Build history of the part. All positions in model axes, mm. Give positions to 0.01 mm unless a question says otherwise; leave off trailing zeros. Loops run counter-clockwise (first coordinate to the right, second up) from the corner with the lowest first, then second, coordinate; pieces in that order, holes last. Notation, with made-up numbers: (2.5, -16.5) -> (46.5, -16.5) arc R26 ccw to (46.5, 7.5) -> close; hole circle Ø5 at (85.25, -13). An arc over 180 degrees is marked (long way). Answer in a Markdown table with one row per item. Add a question column.
from build123d import *

# Parameters (mm, degrees)
F0_R     = 67
F0_R_2   = 8
F0_R_3   = 29.5
F1_DEPTH = 5


with BuildPart() as f1:
    # F0 (on Top) → F1 (new body)
    with BuildSketch(Plane.XY):
        Circle(F0_R)
        with Locations((-15.796341, -47.077298)):
            Circle(F0_R_2, mode=Mode.SUBTRACT)
        with Locations((39.546341, -29.09537)):
            Circle(F0_R_2, mode=Mode.SUBTRACT)
        with Locations((-50, 0)):
            Circle(F0_R_2, mode=Mode.SUBTRACT)
        with Locations((-15.796341, 47.077298)):
            Circle(F0_R_2, mode=Mode.SUBTRACT)
        Circle(F0_R_3, mode=Mode.SUBTRACT)
        with Locations((39.546341, 29.09537)):
            Circle(F0_R_2, mode=Mode.SUBTRACT)
    extrude(amount=F1_DEPTH)


solid = f1.part
(1) Saw through at D-D, the plane y = 33. List the corners of the cut face in (x, z).
(2) Wall check: line 1 along Y through (x, z) = (0, 1.3); line 2 along X through (y, z) = (-2.5, 0.2); line 3 along Y through (x, z) = (-20, 0.8). Give the ranges that are in metal, low to high. Write a range as from..to.
(3) Two-plate mould, pull along X, no slides. Class faces 1 (the cylindrical face through (-17.531, -54.887, 2.465)), 2 (the flat face through (14, -29, 5)), 3 (the cylindrical face through (-14.524, -65.407, 2.465)): released by +X, released by -X, zero draft, split by the parting line, or undercut.
(4) Flat gauge pins, fed straight in: pin 1 Ø2 at (y, z) = (-22, 4) entering from +X; pin 2 Ø9.5 at (x, y) = (-50, 0) entering from -Z; pin 3 Ø3 at (y, z) = (40.5, 1) entering from +X; pin 4 Ø2 at (x, z) = (5, 1) entering from -Y. Where does each tip first touch, or does it go through?
(5) Saw through at C-C, the plane x = -19.5. List the corners of the cut face in (y, z), then the cut area to 3 significant figures.
(6) Saw through at A-A, the plane y = 0. List the corners of the cut face in (x, z).
(7) Saw through at B-B, the plane x = 0. List the corners of the cut face in (y, z).
Worked answers:
| question | item | result |
|---|---|---|
| 1 | outline | (-58.31, 0) -> (32.56, 0) -> (32.56, 5) -> (-58.31, 5) -> close; (46.53, 0) -> (58.31, 0) -> (58.31, 5) -> (46.53, 5) -> close |
| 2 | line 1 | -67..-29.5, 29.5..67 |
| 2 | line 2 | -66.95..-57.6, -42.4..-29.39, 29.39..66.95 |
| 2 | line 3 | -63.95..-53.88, -40.27..-21.69, 21.69..40.27, 53.88..63.95 |
| 3 | face 1 | undercut |
| 3 | face 2 | zero draft |
| 3 | face 3 | split by the parting line |
| 4 | pin 1 | x = 63.62 |
| 4 | pin 2 | through |
| 4 | pin 3 | x = 54.48 |
| 4 | pin 4 | y = -66.88 |
| 5 | outline | (-64.1, 0) -> (-54.17, 0) -> (-54.17, 5) -> (-64.1, 5) -> close; (-39.99, 0) -> (-22.14, 0) -> (-22.14, 5) -> (-39.99, 5) -> close; (22.14, 0) -> (39.99, 0) -> (39.99, 5) -> (22.14, 5) -> close; (54.17, 0) -> (64.1, 0) -> (64.1, 5) -> (54.17, 5) -> close |
| 5 | area | 278 mm^2 |
| 6 | outline | (-67, 0) -> (-58, 0) -> (-58, 5) -> (-67, 5) -> close; (-42, 0) -> (-29.5, 0) -> (-29.5, 5) -> (-42, 5) -> close; (29.5, 0) -> (67, 0) -> (67, 5) -> (29.5, 5) -> close |
| 7 | outline | (-67, 0) -> (-29.5, 0) -> (-29.5, 5) -> (-67, 5) -> close; (29.5, 0) -> (67, 0) -> (67, 5) -> (29.5, 5) -> close |
